Answer from the drawing. Dimensions are ordinates in mm from the lowest x, y and z of the part. Coordinates: 2 decimals unless noted, no trailing zeros. Order: outer loops, then holes, each group sorted by start corner. A loop starts at its lowest first (then second) coordinate and runs counter-clockwise, first axis right, second up. Notation, with made-up numbers: (-31.5, -39) -> (19.5, -39) arc R11 cw to (19.5, -20) -> close; hole circle Ø7 at (-18.5, 86.25). An arc over 180 degrees is marked (long way). Answer in a Markdown table with one row per item.
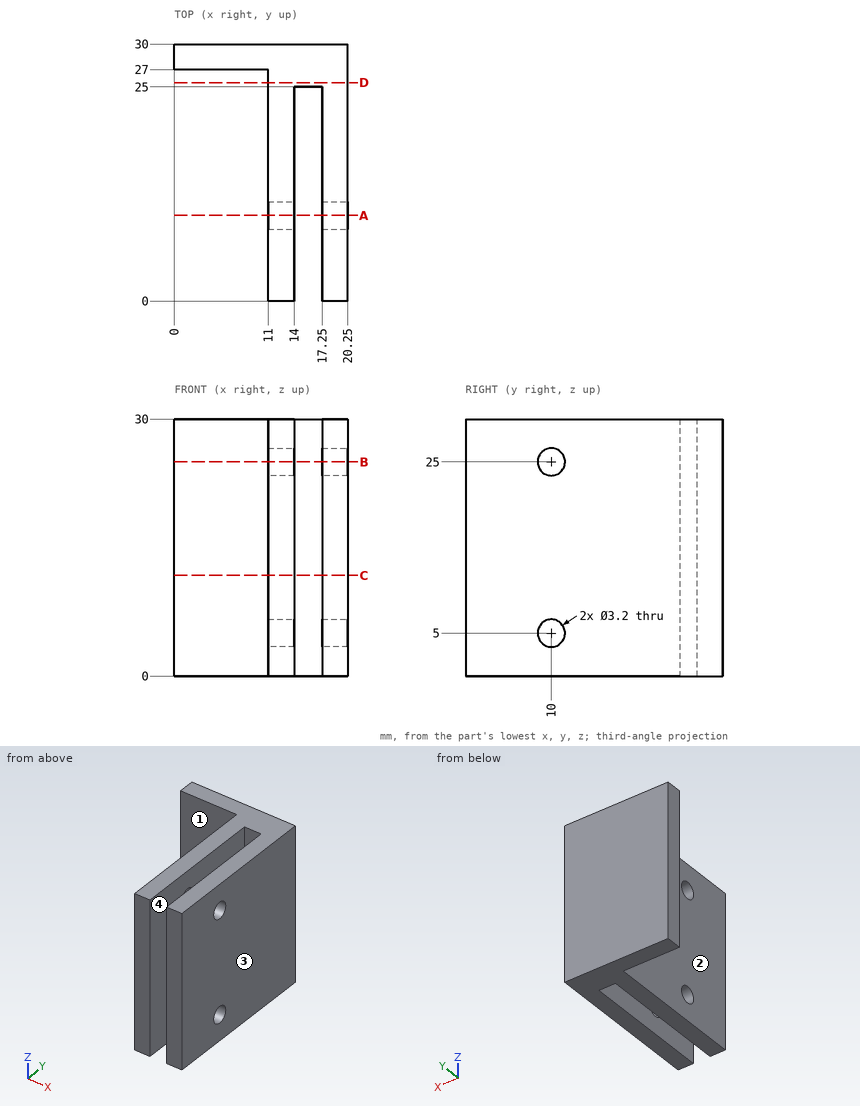
Q1. For a pull along X with two mould halves and no side action, classify the marked faces 1, 2, 3 and 4 as pulls with the +X half, pulls with the -X half, needs draft (parallel to the pull), parting line crosses it, or undercut.
Outcome:
| item | result |
|---|---|
| face 1 | needs draft |
| face 2 | pulls with the -X half |
| face 3 | pulls with the +X half |
| face 4 | undercut |
Q2. The part is cut by section B-B (z = 25). Write down the section's boundary in (x, y), then the cut area to 3 significant figures.
Outcome:
| item | result |
|---|---|
| outline | (0, 27) -> (11, 27) -> (11, 11.6) -> (14, 11.6) -> (14, 25) -> (17.25, 25) -> (17.25, 11.6) -> (20.25, 11.6) -> (20.25, 30) -> (0, 30) -> close; (11, 0) -> (14, 0) -> (14, 8.4) -> (11, 8.4) -> close; (17.25, 0) -> (20.25, 0) -> (20.25, 8.4) -> (17.25, 8.4) -> close |
| area | 210 mm² |
Q3. Consider line 1 (X direction, y = 4, z = 20.5); line 2 (Y direction, x = 17.9, z = 25); line 3 (X direction, y = 26.75, z = 25.75). Determine where each line is inside the solid, lowest interval first.
Outcome:
| item | result |
|---|---|
| line 1 | 11 to 14, 17.25 to 20.25 |
| line 2 | 0 to 8.4, 11.6 to 30 |
| line 3 | 11 to 20.25 |
Q4. The part is cut by section D-D (y = 25.5). Write down the section's boundary in (x, z).
Outcome:
| item | result |
|---|---|
| outline | (11, 0) -> (20.25, 0) -> (20.25, 30) -> (11, 30) -> close |
Q5. The part is cut by section A-A (y = 10). Write down the section's boundary in (x, z).
Outcome:
| item | result |
|---|---|
| outline | (11, 0) -> (14, 0) -> (14, 3.4) -> (11, 3.4) -> close; (11, 6.6) -> (14, 6.6) -> (14, 23.4) -> (11, 23.4) -> close; (11, 26.6) -> (14, 26.6) -> (14, 30) -> (11, 30) -> close; (17.25, 0) -> (20.25, 0) -> (20.25, 3.4) -> (17.25, 3.4) -> close; (17.25, 6.6) -> (20.25, 6.6) -> (20.25, 23.4) -> (17.25, 23.4) -> close; (17.25, 26.6) -> (20.25, 26.6) -> (20.25, 30) -> (17.25, 30) -> close |
Q6. The part is cut by section C-C (z = 11.75). Write down the section's boundary in (x, y).
Outcome:
| item | result |
|---|---|
| outline | (0, 27) -> (11, 27) -> (11, 0) -> (14, 0) -> (14, 25) -> (17.25, 25) -> (17.25, 0) -> (20.25, 0) -> (20.25, 30) -> (0, 30) -> close |
Q7. Given pin 1 (2.5 mm diameter, centred on x = 15.5, z = 9.5, fed in from -Y); pin 2 (13.5 mm diameter, centred on y = 12.5, z = 19.5, fed in from -X), each flat-ended and moving along its own axis, determine where each tip first touches the part or whether it passes through.
Outcome:
| item | result |
|---|---|
| pin 1 | y = 25 |
| pin 2 | x = 11 |
